Here's how the part is built. I have some questions about the finished solid (model axes, mm). Face numbers are marked on the shaded views. A direction names the side the tool comes from. Round coordinates to 2 decimals unless told otherwise and drop trailing zeros. Order: outer loops, then holes, each group sorted by start corner. A loop starts at its lowest first (then second) coordinate and runs counter-clockwise, first axis right, second up.
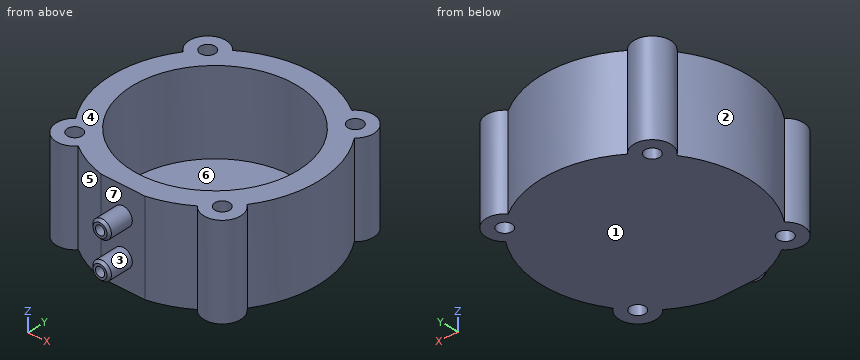
```python
from build123d import *

# Parameters (mm, degrees)
F1_DEPTH  = 20
F2_R      = 1.6
F3_DEPTH  = 20.001
F4_R      = 18
F5_DEPTH  = 18
F6_R      = 2
F7_DEPTH  = 5.5
F9_R      = 1
F10_DEPTH = 25
F11_R     = 1
F12_DEPTH = 25
F13_SIZE  = 0.5


with BuildPart() as f1:
    # F0 (on Top) → F1 (new body)
    with BuildSketch(Plane.XY):
        with BuildLine():
            ThreePointArc((18.475718, 12.841256), (18.73833, 18.73833), (12.841256, 18.475718))
            ThreePointArc((12.841256, 18.475718), (0, 22.5), (-12.841256, 18.475718))
            ThreePointArc((-12.841256, 18.475718), (-18.73833, 18.73833), (-18.475718, 12.841256))
            ThreePointArc((-18.475718, 12.841256), (-22.5, 0), (-18.475718, -12.841256))
            ThreePointArc((-18.475718, -12.841256), (-18.73833, -18.73833), (-12.841256, -18.475718))
            ThreePointArc((-12.841256, -18.475718), (-8.954225, -20.641508), (-4.716991, -22))
            Line((-4.716991, -22), (4.716991, -22))
            ThreePointArc((4.716991, -22), (8.954225, -20.641508), (12.841256, -18.475718))
            ThreePointArc((12.841256, -18.475718), (18.73833, -18.73833), (18.475718, -12.841256))
            ThreePointArc((18.475718, -12.841256), (22.5, 0), (18.475718, 12.841256))
        make_face()
    extrude(amount=F1_DEPTH)

    # F2 (on face) → F3 (cut, through all)
    with BuildSketch(Plane.XY.offset(20)):
        with Locations((-15.909903, 15.909903)):
            Circle(F2_R)
        with Locations((15.909903, 15.909903)):
            Circle(F2_R)
        with Locations((15.909903, -15.909903)):
            Circle(F2_R)
        with Locations((-15.909903, -15.909903)):
            Circle(F2_R)
    extrude(amount=-F3_DEPTH, mode=Mode.SUBTRACT)

    # F4 (on face) → F5 (cut)
    with BuildSketch(Plane.XY.offset(20)):
        Circle(F4_R)
    extrude(amount=-F5_DEPTH, mode=Mode.SUBTRACT)

    # F6 (on face) → F7 (join)
    with BuildSketch(Plane.XZ.offset(22)):
        with Locations((0, 14)):
            Circle(F6_R)
        with Locations((0, 6)):
            Circle(F6_R)
    extrude(amount=F7_DEPTH)

    # F9 (on face) → F10 (cut)
    with BuildSketch(Plane.XZ.offset(27.5)):
        with Locations((0, 6)):
            Circle(F9_R)
    extrude(amount=-F10_DEPTH, mode=Mode.SUBTRACT)

    # F11 (on face) → F12 (cut)
    with BuildSketch(Plane.XZ.offset(27.5)):
        with Locations((0, 14)):
            Circle(F11_R)
    extrude(amount=-F12_DEPTH, mode=Mode.SUBTRACT)

    # F13
    f13_edges = [f1.edges().sort_by_distance(p)[0] for p in [
        (-2, -27.5, 14),
        (-2, -27.5, 6),
    ]]
    chamfer(f13_edges, length=F13_SIZE)


solid = f1.part
```
1. On a 3-axis mill with a long thin cutter (end or side, diameter ignored), from which of +Z, -Z, +X, -X, +Y, -Y can I reach the whole of each face in a straight line? I mean the marked faces 4, 5, 6 and 7. Say none if no direction works.
Evaluation:
face 4: +Z, +X, -X, +Y, -Y
face 5: +Z, -Z, -Y
face 6: +Z
face 7: -Y
2. I'm going to push flat-ended pins straight in: P1, Ø1.2, axis at x = 0, z = 14, coming from the +Y side; P2, Ø7.5, axis at x = -1.5, z = 13.5, coming from the -Y side; P3, Ø6, axis at x = -10.5, y = 3, coming from the +Z side; P4, Ø1.5, axis at x = -14.5, z = 4.5, coming from the +Y side. Where does each tip first touch, or does it pass through?
Evaluation:
P1: stops at y = 22.5
P2: stops at y = -27.5
P3: stops at z = 2
P4: stops at y = 19.86
3. If we mould it in two halves opening along Z, with no side actions, what happens to the marked faces 1, 2 and 3? For each: released by +Z, released by -Z, zero draft, split by the parting line, or undercut.
Evaluation:
face 1: released by -Z
face 2: zero draft
face 3: undercut
4. If we section it at B-B, the plane x = 0: Write out the boundary of the cut face in (y, z), and give its area (4 significant figures).
Evaluation:
outline: (-27.5, 4.5) - (-27, 4) - (-22, 4) - (-22, 0) - (22.5, 0) - (22.5, 20) - (18, 20) - (18, 2) - (-18, 2) - (-18, 5) - (-27.5, 5) - close; (-27.5, 7) - (-18, 7) - (-18, 13) - (-27.5, 13) - (-27.5, 12.5) - (-27, 12) - (-22, 12) - (-22, 8) - (-27, 8) - (-27.5, 7.5) - close; (-27.5, 15) - (-18, 15) - (-18, 20) - (-22, 20) - (-22, 16) - (-27, 16) - (-27.5, 15.5) - close
area: 247.5 mm2
5. If we section it at C-C, the plane y = -16.5: Write out the boundary of the cut face in (x, z).
Evaluation:
outline: (-19.87, 0) - (-17.4, 0) - (-17.4, 20) - (-19.87, 20) - close; (-14.42, 0) - (14.42, 0) - (14.42, 20) - (7.19, 20) - (7.19, 2) - (-7.19, 2) - (-7.19, 20) - (-14.42, 20) - close; (17.4, 0) - (19.87, 0) - (19.87, 20) - (17.4, 20) - close
6. If we section it at D-D, the plane z = 6: Write out the boundary of the cut face in (x, y).
Evaluation:
outline: (-18.48, -12.84) arc R4 ccw (long way) to (-12.84, -18.48) arc R22.5 ccw to (-4.72, -22) - (-2, -22) - (-2, -27) - (-1.5, -27.5) - (-1, -27.5) - (-1, -17.97) arc R18 cw (long way) to (1, -17.97) - (1, -27.5) - (1.5, -27.5) - (2, -27) - (2, -22) - (4.72, -22) arc R22.5 ccw to (12.84, -18.48) arc R4 ccw (long way) to (18.48, -12.84) arc R22.5 ccw to (18.48, 12.84) arc R4 ccw (long way) to (12.84, 18.48) arc R22.5 ccw to (-12.84, 18.48) arc R4 ccw (long way) to (-18.48, 12.84) arc R22.5 ccw to start; hole circle Ø3.2 at (-15.91, -15.91); hole circle Ø3.2 at (-15.91, 15.91); hole circle Ø3.2 at (15.91, -15.91); hole circle Ø3.2 at (15.91, 15.91)
7. I need wall thicknesses on probe 1 along X at (y, z) = (16, 13.25); probe 2 along X at (y, z) = (-19.5, 18.5); probe 3 along X at (y, z) = (15.5, 2.25). Which ranges of each line are inside material? Lowest first, please.
Evaluation:
probe 1: x = -19.91 to -17.51, -14.31 to -8.25, 8.25 to 14.31, 17.51 to 19.91
probe 2: x = -17.67 to -14.15, -11.22 to 11.22, 14.15 to 17.67
probe 3: x = -19.89 to -17.46, -14.36 to -9.15, 9.15 to 14.36, 17.46 to 19.89
8. If we section it at A-A, the plane y = 0: Write out the boundary of the cut face in (x, z).
Evaluation:
outline: (-22.5, 0) - (22.5, 0) - (22.5, 20) - (18, 20) - (18, 2) - (-18, 2) - (-18, 20) - (-22.5, 20) - close
